Drawing for the job (mm, zero at the part's lowest x, y, z). Give positions to 0.01 mm unless a question says otherwise; leave off trailing zeros. Order: outer loops, then holes, each group sorted by start corner. A loop starts at its lowest first (then second) coordinate and runs counter-clockwise, first axis right, second up. Notation, with made-up numbers: M 87,-28.5 L 99,-28.5 A16 cw 99,-2.5 Z; hole C -17,34.5 d4. An arc over 180 degrees is marked long. Answer as a JSON object with one key per item and string values.
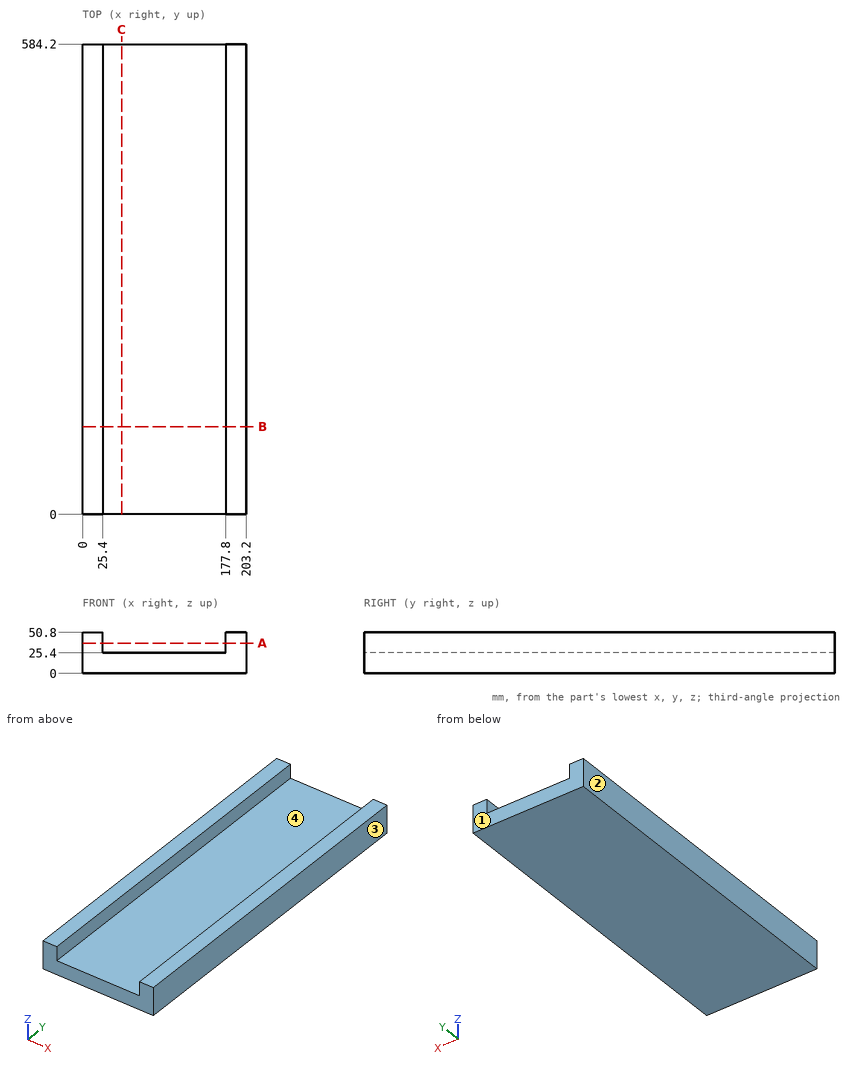
1. Probe line 1 along X through (y, z) = (68, 35); line 2 along Z through (x, y) = (25.5, 486.5). List the from-to ranges inside material, lowest first.
Worked answers:
{"line 1": "x = 0 to 25.4, 177.8 to 203.2", "line 2": "z = 0 to 25.4"}
2. Cut at C-C on x = 48.5. Give the cut face in (y, z), plus the area to 3 significant figures.
Worked answers:
{"outline": "M 0,0 L 584.2,0 L 584.2,25.4 L 0,25.4 Z", "area": "14,800 mm^2"}
3. Cut at B-B on y = 109. Give the cut face in (x, z), plus the area to 3 significant figures.
Worked answers:
{"outline": "M 0,0 L 203.2,0 L 203.2,50.8 L 177.8,50.8 L 177.8,25.4 L 25.4,25.4 L 25.4,50.8 L 0,50.8 Z", "area": "6,450 mm^2"}
4. Cut at A-A on z = 37.5. Give the cut face in (x, y).
Worked answers:
{"outline": "M 0,0 L 25.4,0 L 25.4,584.2 L 0,584.2 Z; M 177.8,0 L 203.2,0 L 203.2,584.2 L 177.8,584.2 Z"}
5. Pin check, flat tips, straight feed: P1, Ø12, axis at x = 168.5, y = 324.5, coming from the +Z side; P2, Ø6, axis at x = 22, z = 10, coming from the -Y side. Stop position of each tip, or through.
Worked answers:
{"P1": "stops at z = 25.4", "P2": "stops at y = 0"}
6. Two-plate mould, pull along X, no slides. Class the marked faces 1, 2, 3 and 4: +X half, -X half, draft (parallel to the pull), parting line (faces both ways), or undercut.
Worked answers:
{"face 1": "draft", "face 2": "-X half", "face 3": "+X half", "face 4": "undercut"}
